Read the model definition and answer for the solid it produces. Units are mm, in the model's axes. Face numbers are marked on the shaded views. A direction names the side the tool comes from. Coordinates: 2 decimals unless noted, no trailing zeros. Order: outer loops, then holes, each group sorted by start corner. A loop starts at its lowest first (then second) coordinate and runs counter-clockwise, first axis right, second up. Notation, with made-up numbers: (-7, 57) - (19, 57) arc R20 ccw to (19, 85) - close; hole circle Ø3 at (33, 0.5). An arc over 180 degrees is marked (long way). Write item = value, one per line.
from build123d import *

# Parameters (mm, degrees)
CROQUIS1_W              = 36
CROQUIS1_H              = 7
CROQUIS1_R              = 2.6
SALIENTE_EXTRUIR1_DEPTH = 10
CORTAR_EXTRUIR1_DEPTH   = 7
CROQUIS4_W              = 11.4
CROQUIS4_H              = 10
SALIENTE_EXTRUIR2_DEPTH = 5
REDONDEO1_R             = 2
CROQUIS5_W              = 11.4
CROQUIS5_H              = 10
CROQUIS5_R              = 3.25
SALIENTE_EXTRUIR3_DEPTH = 2.3


with BuildPart() as part:
    # Croquis1 → Saliente-Extruir1 (new body)
    with BuildSketch(Plane.XY):
        with Locations((-28.016694491, 12.37804878)):
            Rectangle(CROQUIS1_W, CROQUIS1_H)
        with Locations((-41.766694491, 12.37804878)):
            Circle(CROQUIS1_R, mode=Mode.SUBTRACT)
        with Locations((-14.266694491, 12.37804878)):
            Circle(CROQUIS1_R, mode=Mode.SUBTRACT)
    extrude(amount=SALIENTE_EXTRUIR1_DEPTH)

    # Croquis2 → Cortar-Extruir1 (cut)
    with BuildSketch(Plane.XZ.offset(-8.87804878)):
        Polygon((-29.724687257, 5), (-32.120690874, 9.15), (-36.912698108, 9.15), (-39.308701725, 5), (-36.912698108, 0.85), (-32.120690874, 0.85), align=None)
    extrude(amount=-CORTAR_EXTRUIR1_DEPTH, mode=Mode.SUBTRACT)

    # Croquis4 → Saliente-Extruir2 (add)
    with BuildSketch(Plane.XZ.offset(-8.87804878)):
        with Locations((-34.516694491, 5)):
            Rectangle(CROQUIS4_W, CROQUIS4_H)
        Polygon((-29.724687257, 5), (-32.120690874, 9.15), (-36.912698108, 9.15), (-39.308701725, 5), (-36.912698108, 0.85), (-32.120690874, 0.85), align=None, mode=Mode.SUBTRACT)
    extrude(amount=SALIENTE_EXTRUIR2_DEPTH)

    # Redondeo1
    redondeo1_edges = [part.edges().sort_by_distance(p)[0] for p in [
        (-10.016694491, 15.87804878, 5),
        (-10.016694491, 8.87804878, 5),
        (-46.016694491, 8.87804878, 5),
        (-46.016694491, 15.87804878, 5),
    ]]
    fillet(redondeo1_edges, radius=REDONDEO1_R)

    # Croquis5 → Saliente-Extruir3 (add)
    with BuildSketch(Plane.XZ.offset(-3.87804878)):
        with Locations((-34.516694491, 5)):
            Rectangle(CROQUIS5_W, CROQUIS5_H)
        with Locations(Location((-34.516694491, 5, 0), (0, 0, 270))):
            Circle(CROQUIS5_R, mode=Mode.SUBTRACT)
    extrude(amount=SALIENTE_EXTRUIR3_DEPTH)


solid = part.part
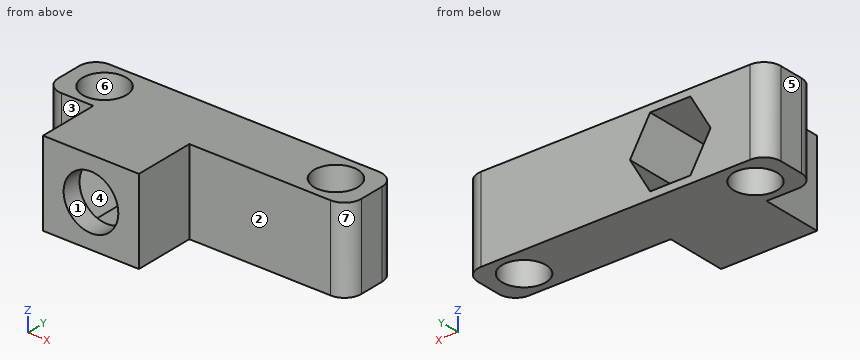
1) For the marked faces 1, 2, 3 and 4, determine the directions among +Z, -Z, +X, -X, +Y, -Y from which every point of the face is accessible in a straight line to the end or side of a thin tool.
Returned:
face_1 = +Y, -Y
face_2 = +Z, -Z, +X, -Y
face_3 = +Z, -Z, -X, -Y
face_4 = +Y
2) Flat-ended cylindrical pins translate along their axes: pin 1 Ø3.5 at (y, z) = (3.5, 6) entering from -X; pin 2 Ø6 at (x, z) = (-34.52, 5) entering from +Y; pin 3 Ø3 at (x, z) = (-23, 6) entering from -Y; pin 4 Ø6 at (y, z) = (6.5, 3) entering from +X. Find the tip coordinate at first contact, or state that the pin passes through.
Returned:
pin_1 = -40.22
pin_2 = through
pin_3 = 8.88
pin_4 = -10.57
3) Straight lines are drawn through the part: line 1 along Z through (x, y) = (-32.5, 6); line 2 along X through (y, z) = (13.5, 1); line 3 along X through (y, z) = (13.5, 0.75). For each, find the intervals that lie inside material, in ascending order. Write a range as from..to.
Returned:
line_1 = 0..0.85, 9.15..10
line_2 = -46.02..-44.11, -39.42..-37, -32.03..-16.61, -11.92..-10.02
line_3 = -46.02..-44.11, -39.42..-16.61, -11.92..-10.02
4) The part is cut by section A-A (z = 6.75). Determine the outline of the cut face in (x, y).
Returned:
outline = (-46.02, 10.88) arc R2 ccw to (-44.02, 8.88) - (-40.22, 8.88) - (-40.22, 1.58) - (-37.26, 1.58) - (-37.26, 3.88) - (-38.3, 3.88) - (-38.3, 15.88) - (-44.02, 15.88) arc R2 ccw to (-46.02, 13.88) - close; (-31.78, 1.58) - (-28.82, 1.58) - (-28.82, 8.88) - (-12.02, 8.88) arc R2 ccw to (-10.02, 10.88) - (-10.02, 13.88) arc R2 ccw to (-12.02, 15.88) - (-30.74, 15.88) - (-30.74, 3.88) - (-31.78, 3.88) - close; hole circle Ø5.2 at (-41.77, 12.38); hole circle Ø5.2 at (-14.27, 12.38)
5) The part is cut by section C-C (y = 12). Determine the outline of the cut face in (x, z).
Returned:
outline = (-46.02, 0) - (-44.34, 0) - (-44.34, 10) - (-46.02, 10) - close; (-39.19, 0) - (-16.84, 0) - (-16.84, 10) - (-39.19, 10) - (-39.19, 5.2) - (-36.91, 9.15) - (-32.12, 9.15) - (-29.72, 5) - (-32.12, 0.85) - (-36.91, 0.85) - (-39.19, 4.8) - close; (-11.69, 0) - (-10.02, 0) - (-10.02, 10) - (-11.69, 10) - close
6) The part is cut by section B-B (y = 8.5). Determine the outline of the cut face in (x, z).
Returned:
outline = (-40.22, 0) - (-28.82, 0) - (-28.82, 10) - (-40.22, 10) - close; hole (-39.31, 5) - (-36.91, 0.85) - (-32.12, 0.85) - (-29.72, 5) - (-32.12, 9.15) - (-36.91, 9.15) - close
7) Determine the mould class of the marked faces 5, 6 and 7 for opening direction Y: pulls with the +Y half, pulls with the -Y half, needs draft (parallel to the pull), parting line crosses it, or undercut.
Returned:
face_5 = needs draft
face_6 = undercut
face_7 = pulls with the -Y half
8) The part is cut by section D-D (x = -14). Determine the outline of the cut face in (y, z), and give its area (3 significant figures).
Returned:
outline = (8.88, 0) - (9.79, 0) - (9.79, 10) - (8.88, 10) - close; (14.96, 0) - (15.88, 0) - (15.88, 10) - (14.96, 10) - close
area = 18.3 mm^2
